Here's how the part is built. I have some questions about the finished solid (model axes, mm). Face numbers are marked on the shaded views. Round coordinates to 2 decimals unless told otherwise and drop trailing zeros. Write each loop counter-clockwise with the first axis right and the second up, starting at its lowest first coordinate (ties: lowest second). Pieces come first, ordered by that corner, then holes. Notation, with made-up numbers: (28.5, -37) -> (85.5, -37) arc R20 ccw to (85.5, -16) -> close; hole circle Ø9 at (3, 32). An arc over 180 degrees is marked (long way). Put each result on its own line as item: value. Start each with the question number.
1) If I drill on line 1 along X through (y, z) = (32, 0); line 2 along Y through (x, z) = (7.5, -4), over which ranges is the centre line in solid material (lowest first)? Write a range as [from, to].
2) I want a section at A-A, the plane z = 0. List the corners of the cut face in (x, y) for me.
3) I want a section at B-B, the plane x = 0. List the corners of the cut face in (y, z) for me.
4) I want a section at D-D, the plane z = -7.75. List the corners of the cut face in (x, y) for me, then the cut area to 3 significant figures.
5) Will these pins go through, and if not, where does the flat tip stop? P1, Ø1.5, axis at x = 6.5, y = 14.5, coming from the +Z side; P2, Ø8, axis at y = 53, z = 5, coming from the +X side; P3, Ø1.5, axis at y = 24.5, z = -6, coming from the -X side; P4, Ø8, axis at x = 0, z = 0, coming from the +Y side.
6) We'd pull the mould along Y, two halves only. Please class the marked faces 1, 2 and 3: released by +Y, released by -Y, zero draft, split by the parting line, or undercut.
7) I want a section at C-C, the plane y = 6. List the corners of the cut face in (x, z) for me.
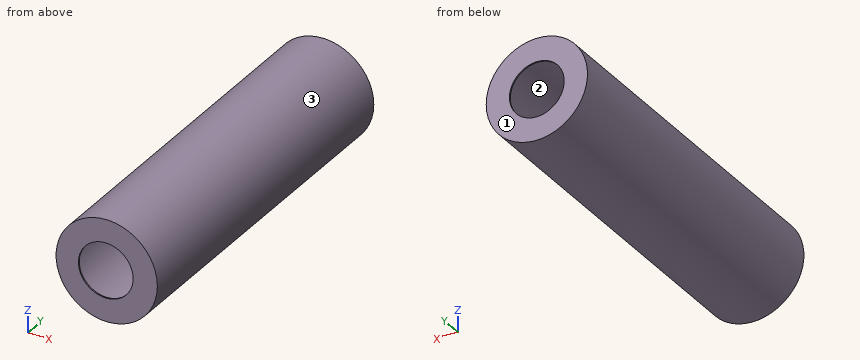
from build123d import *

# Parameters (mm, degrees)
SKETCH1_R           = 9.25
SKETCH1_R_2         = 9
BOSS_EXTRUDE1_DEPTH = 65.1
SKETCH2_R           = 9.25
SKETCH2_R_2         = 5
BOSS_EXTRUDE2_DEPTH = 0.25
SKETCH3_R           = 9.25
SKETCH3_R_2         = 5
BOSS_EXTRUDE3_DEPTH = 0.25


with BuildPart() as part:
    # Sketch1 → Boss-Extrude1 (new body)
    with BuildSketch(Plane(origin=(0, 0, 0), x_dir=(1, 0, 0), z_dir=(0, 1, 0))):
        Circle(SKETCH1_R)
        Circle(SKETCH1_R_2, mode=Mode.SUBTRACT)
    extrude(amount=BOSS_EXTRUDE1_DEPTH)

    # Sketch2 → Boss-Extrude2 (add)
    with BuildSketch(Plane(origin=(0, 65.1, 0), x_dir=(1, 0, 0), z_dir=(0, 1, 0))):
        Circle(SKETCH2_R)
        Circle(SKETCH2_R_2, mode=Mode.SUBTRACT)
    extrude(amount=BOSS_EXTRUDE2_DEPTH)

    # Sketch3 → Boss-Extrude3 (add)
    with BuildSketch(Plane.XZ):
        Circle(SKETCH3_R)
        with Locations((-0.172396434, 0)):
            Circle(SKETCH3_R_2, mode=Mode.SUBTRACT)
    extrude(amount=BOSS_EXTRUDE3_DEPTH)


solid = part.part
Findings:
1. line 1: x = [-9.25, -9], [9, 9.25]
1. line 2: y = [-0.25, 0], [65.1, 65.35]
2. outline: (-9.25, -0.25) -> (-5.17, -0.25) -> (-5.17, 0) -> (-9, 0) -> (-9, 65.1) -> (-5, 65.1) -> (-5, 65.35) -> (-9.25, 65.35) -> close; (4.83, -0.25) -> (9.25, -0.25) -> (9.25, 65.35) -> (5, 65.35) -> (5, 65.1) -> (9, 65.1) -> (9, 0) -> (4.83, 0) -> close
3. outline: (-0.25, -9.25) -> (65.35, -9.25) -> (65.35, -5) -> (65.1, -5) -> (65.1, -9) -> (0, -9) -> (0, -5) -> (-0.25, -5) -> close; (-0.25, 5) -> (0, 5) -> (0, 9) -> (65.1, 9) -> (65.1, 5) -> (65.35, 5) -> (65.35, 9.25) -> (-0.25, 9.25) -> close
4. outline: (-5.05, -0.25) -> (5.05, -0.25) -> (5.05, 65.35) -> (-5.05, 65.35) -> close; hole (-4.58, 0) -> (4.58, 0) -> (4.58, 65.1) -> (-4.58, 65.1) -> close
4. area: 66.8 mm2
5. P1: stops at z = 7.25
5. P2: stops at x = 9.2
5. P3: stops at x = -7.62
5. P4: passes through
6. face 1: released by +Y
6. face 2: undercut
6. face 3: zero draft
7. outline: circle Ø18.5 at (0, 0); hole circle Ø18 at (0, 0)
